Design review of the part built by this model. Coordinates are the model's own, in mm. A direction names the side the tool comes from. Round coordinates to 2 decimals unless told otherwise and drop trailing zeros. Order: outer loops, then holes, each group sorted by start corner. A loop starts at its lowest first (then second) coordinate and runs counter-clockwise, first axis right, second up. Notation, with made-up numbers: (3.5, 7) - (61.5, 7) arc R17 ccw to (61.5, 11) - close; hole circle Ø7 at (55.25, 57.5). An arc over 180 degrees is marked (long way). Answer as a JSON object with one key per item and string values. Group by question number.
from build123d import *

# Parameters (mm, degrees)
F0_W     = 152.4
F0_H     = 76.2
F1_DEPTH = 25.4
F2_R     = 12.7
F3_DEPTH = 12.7
F4_SIZE  = 2.54
F7_R     = 2.53999


# Not quite as in the source:
# - a fillet or chamfer is up to 0.001 mm smaller than in the source, because OpenCascade refuses the exact size


with BuildPart() as f1:
    # F0 (on Top) → F1 (new body)
    with BuildSketch(Plane.XY):
        Rectangle(F0_W, F0_H)
    extrude(amount=F1_DEPTH)

    # F2 (on face) → F3 (cut)
    with BuildSketch(Plane.XY.offset(25.4)):
        with Locations((57.15, -19.05)):
            Circle(F2_R)
        with Locations((-57.15, -19.05)):
            Circle(F2_R)
        with Locations((-57.15, 19.05)):
            Circle(F2_R)
        with Locations((57.15, 19.05)):
            Circle(F2_R)
    extrude(amount=-F3_DEPTH, mode=Mode.SUBTRACT)

    # F4
    f4_edges = [f1.edges().sort_by_distance(p)[0] for p in [
        (0, -38.1, 25.4),
        (76.2, 0, 25.4),
        (0, 38.1, 25.4),
        (-76.2, 0, 25.4),
    ]]
    chamfer(f4_edges, length=F4_SIZE)

    # F5 (on Front) → F6 (revolve)
    with BuildSketch(Plane.XZ):
        Polygon((0, 63.5), (0, 25.4), (19.05, 25.4), (19.05, 38.1), (16.51, 38.1), (16.51, 50.8), (19.05, 50.8), (19.05, 63.5), align=None)
    revolve(axis=Axis((0, 0, 44.45), (0, 0, 1)))

    # F7 (radius 2.54 in the source; OpenCascade refuses exactly that, so slightly less here)
    f7_edges = [f1.edges().sort_by_distance(p)[0] for p in [
        (-16.51, 0, 38.1),
        (-19.05, 0, 25.4),
        (-16.51, 0, 50.8),
        (-19.05, 0, 63.5),
    ]]
    fillet(f7_edges, radius=F7_R)


solid = f1.part
1. Take a section at A-A, the plane x = -57.15. Give the boundary of the cut face in (y, z).
2. Mouldability with a two-part tool opening along X and no side actions: class faces 4 (the cylindrical face through (-45.418, 14.186, 19.139)), 5 (the flat face through (76.2, -1, 11)), 6 (the flat face through (-1, -38.1, 11)) as pulls with the +X half, pulls with the -X half, needs draft (parallel to the pull), parting line crosses it, or undercut.
3. Tool access review of faces 1 (the cylindrical face through (15.748, 4.959, 44.503)), 2 (the flat face through (0, 0, 63.5)), 3 (the flat face through (57, -19, 12.7)): name each direction out of +Z, -Z, +X, -X, +Y, -Y from which nothing blocks a thin tool from reaching the whole face with its end or side.
4. Clearance check with flat-ended pins moving along their axes: P1, Ø12.5, axis at x = -53.5, y = 14, coming from the +Z side; P2, Ø5, axis at x = 28, y = -21.5, coming from the +Z side. State where each tip first meets the part, or that it passes through.
5. To check wall thickness, follow line 1 (Y direction, x = 57.15, z = 16); line 2 (X direction, y = -19, z = 20); line 3 (X direction, y = -22.5, z = 17.5). State the ranges of each line that lie inside material, in increasing order. Write a range as from..to.
Response values:
{
 "1": {"outline": "(-38.1, 0) - (38.1, 0) - (38.1, 22.86) - (35.56, 25.4) - (31.75, 25.4) - (31.75, 12.7) - (6.35, 12.7) - (6.35, 25.4) - (-6.35, 25.4) - (-6.35, 12.7) - (-31.75, 12.7) - (-31.75, 25.4) - (-35.56, 25.4) - (-38.1, 22.86) - close"},
 "2": {"face 4": "undercut", "face 5": "pulls with the +X half", "face 6": "needs draft"},
 "3": {"face 1": "none", "face 2": "+Z, +X, -X, +Y, -Y", "face 3": "+Z"},
 "4": {"P1": "z = 12.7", "P2": "z = 25.4"},
 "5": {"line 1": "-38.1..-31.75, -6.35..6.35, 31.75..38.1", "line 2": "-76.2..-69.85, -44.45..44.45, 69.85..76.2", "line 3": "-76.2..-69.37, -44.93..44.93, 69.37..76.2"}
}
